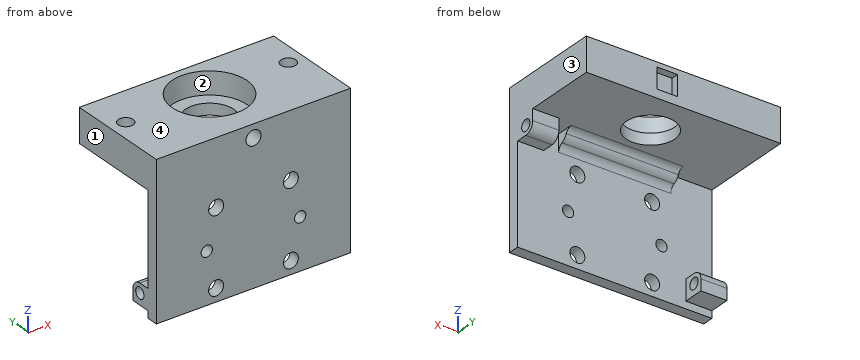
Autodesk Inventor part; units mm, degrees
ref_plane "YZ Plane" through (0, 0, 0) normal (1, 0, 0) x (0, 1, 0)
ref_plane "XZ Plane" through (0, 0, 0) normal (0, 1, 0) x (-1, 0, 0)
ref_plane "XY Plane" through (0, 0, 0) normal (0, 0, 1) x (1, 0, 0)
sketch "Boceto1" plane through (0, 0, 0) normal (0, 0, 1) x (1, 0, 0)
  line L0 (-26, 1.5) -> (26, 1.5)
  line L1 (26, 1.5) -> (26, -1.5)
  line L2 (26, -1.5) -> (-26, -1.5)
  line L3 (-26, -1.5) -> (-26, 1.5)
  line L4 (2.9301, 0) -> (0, 0)
  line L5 (0, 0) -> (0, 1.8389)
  dimension "d0" = 52
  dimension "d1" = 3
extrude "Extrusión1" add sketch "Boceto1" along normal blind 30
sketch "Boceto3" plane through (-26, 1.5, 0) normal (0, 1, 0) x (1, 0, 0)
  line L0 (52, 0) -> (52, -30)
  line L1 (0, -30) -> (52, -30)
  line L2 (52, 0) -> (47, 0)
  line L3 (47, 0) -> (47, -30)
  line L4 (47, -30) -> (52, -30)
  line L5 (52, -30) -> (52, 0)
  line L6 (0, 0) -> (0, -30)
  line L7 (0, 0) -> (5, 0)
  line L8 (5, 0) -> (5, -30)
  line L9 (5, -30) -> (0, -30)
  line L10 (0, -30) -> (0, 0)
  point P0 (26, 0)
  point P1 (5, -30)
  dimension "d4" = 5
  dimension "d5" = 5
extrude "Extrusión2" add sketch "Boceto3" along normal blind 25
sketch "Boceto5" plane through (0, 0, 30) normal (0, 0, 1) x (1, 0, 0)
  line L0 (-26, -1.5) -> (26, -1.5)
  line L1 (-26, -1.5) -> (-26, 26.5)
  line L2 (26, -1.5) -> (-26, -1.5)
  line L3 (-26, -1.5) -> (-26, 26.5)
  line L4 (-26, 26.5) -> (26, 26.5)
  line L5 (26, 26.5) -> (26, -1.5)
  point P0 (0, 0)
extrude "Extrusión4" add sketch "Boceto5" along normal blind 3
sketch "Boceto6" plane through (0, 0, 33) normal (0, 0, 1) x (1, 0, 0)
  circle A0 centre (0, 14.5) radius 6.5
  line L0 (26, -1.5) -> (26, 26.5)
  line L1 (26, 26.5) -> (-26, 26.5)
  line L2 (-26, 26.5) -> (-26, -1.5)
  point P0 (0, 0)
  point P1 (2.0533, 26.5)
  point P2 (-6.2533, 26.5)
  dimension "d12" = 13
  dimension "d13" = 26
  dimension "d14" = 12
  dimension "d38" = 52
extrude "Extrusión5" cut sketch "Boceto6" against normal up to surface (3 mm away)
sketch "Boceto7" plane through (-21, 1.5, 0) normal (0, 1, 0) x (1, 0, 0)
  circle A0 centre (33.5, -11.5916) radius 1.5
  circle A1 centre (8.5, -11.5916) radius 1.5
  line L0 (21, 0) -> (21, -4.282)
  line L1 (47, -33) -> (-5, -33)
  dimension "d17" = 25
  dimension "d18" = 12.5
  dimension "d19" = 3
  dimension "d20" = 3
  dimension "d68" = 21.4084
extrude "Extrusión6" cut sketch "Boceto7" against normal through all
sketch "Boceto9" plane through (0, 0, 33) normal (0, 0, 1) x (1, 0, 0)
  circle A0 centre (0, 14.5) radius 6.5
  line L0 (-26, 26.5) -> (-26, -1.5)
  line L1 (26, 26.5) -> (-26, 26.5)
  line L2 (26, -1.5) -> (26, 26.5)
  line L3 (-26, -1.5) -> (26, -1.5)
  circle A1 centre (0, 14.5) radius 10
  point P0 (0, 0)
  point P1 (0, 26.5)
  dimension "d32" = 20
extrude "Extrusión8" add sketch "Boceto9" along normal blind 6 contours L1 L2 L3 L0
sketch "Boceto8" plane through (0, 0, 39) normal (0, 0, 1) x (1, 0, 0)
  circle A0 centre (21.75, 15.395) radius 2
  circle A1 centre (-21.75, 15.395) radius 2
  line L0 (26, 26.5) -> (-26, 26.5)
  circle A2 centre (0, 14.5) radius 10
  point P0 (0, 0)
  dimension "d23" = 4
  dimension "d24" = 4
  dimension "d25" = 43.5
  dimension "d35" = 11.105
  dimension "d36" = 11.105
  dimension "d37" = 21.75
extrude "Extrusión7" cut sketch "Boceto8" against normal blind 5 contours A0 | A1
sketch "Boceto10" plane through (-26, 26.5, 0) normal (0, 1, 0) x (1, 0, 0)
  circle A0 centre (30.3, -35) radius 2
  line L0 (52, 0) -> (52, -39)
  line L1 (52, -39) -> (0, -39)
  line L2 (27.55, -32.25) -> (33.05, -32.25)
  line L3 (33.05, -32.25) -> (33.05, -37.75)
  line L4 (33.05, -37.75) -> (27.55, -37.75)
  line L5 (27.55, -37.75) -> (27.55, -32.25)
  line L6 (27.55, -32.25) -> (33.05, -37.75) construction
  line L7 (33.05, -32.25) -> (27.55, -37.75) construction
  point P0 (26, 0)
  dimension "d39" = 21.7
  dimension "d41" = 4
  dimension "d45" = 5.5
  dimension "d46" = 5.5
extrude "Extrusión9" cut sketch "Boceto10" against normal blind 2 contours A0 | L2 L3 L4 L5
sketch "Boceto11" plane through (26, -1.5, 0) normal (1, 0, 0) x (0, 0, -1)
  line L0 (-30, 28) -> (0, 28)
  line L1 (0, 28) -> (-30, 28)
  line L2 (-30, 28) -> (-30, 3)
  line L3 (-30, 3) -> (0, 3)
  line L4 (0, 3) -> (0, 28)
  point P0 (0, 1.5)
  dimension "d47" = 30
  dimension "d48" = 25
extrude "Extrusión10" cut sketch "Boceto11" against normal up to surface (52 mm away)
sketch "Boceto12" plane through (-26, -1.5, 0) normal (0, -1, 0) x (1, 0, 0)
  circle A0 centre (26, 35.5) radius 2
  line L0 (0, 0) -> (0, 39)
  line L1 (52, 0) -> (52, 39)
  line L2 (0, 39) -> (52, 39)
  point P0 (26, 0)
  dimension "d51" = 4
  dimension "d52" = 52
  dimension "d53" = 26
  dimension "d54" = 3.5
extrude "Extrusión11" cut sketch "Boceto12" against normal blind 5
sketch "Boceto13" plane through (26, -1.5, 0) normal (1, 0, 0) x (0, 0, -1)
  line L0 (-30, 3) -> (0, 3)
  line L1 (-24.5, 3) -> (-24.5, 8.5)
  line L2 (-24.5, 3) -> (-19, 3) construction
  line L3 (-24.5, 8.5) -> (-30, 8.5)
  line L4 (-30, 3) -> (-30, 28)
  circle A0 centre (-27, 6) radius 1.5
  point P0 (0, 1.5)
  dimension "d57" = 5.5
  dimension "d58" = 90
  dimension "d59" = 5.5
  dimension "d63" = 3
  dimension "d64" = 3
  dimension "d65" = 3
extrude "Extrusión12" add sketch "Boceto13" against normal blind 7
fillet "Empalme2" radius 2.5 1 edges at (22.5, 7, 24.5)
sketch "Boceto16" plane through (-26, 1.5, 0) normal (0, 1, 0) x (1, 0, 0)
  line L0 (0, -30) -> (0, 0)
  line L1 (0, 0) -> (52, 0)
  line L2 (52, 0) -> (52, 1.908)
  line L3 (52, 1.908) -> (0, 1.908)
  line L4 (0, 1.908) -> (0, 0)
  line L5 (52, 0) -> (52, -24.5)
  point P0 (26, 0)
  dimension "d69" = 1.908
extrude "Extrusión13" add sketch "Boceto16" against normal up to surface (3 mm away)
sketch "Boceto17" plane through (-26, 1.5, 30) normal (0, 1, 0) x (1, 0, 0)
  circle A0 centre (16, 28.408) radius 2
  line L0 (52, 31.908) -> (0, 31.908)
  point P0 (26, 30)
  dimension "d72" = 4
  dimension "d73" = 3.5
  dimension "d82" = 10
extrude "Extrusión14" cut sketch "Boceto17" against normal through all
pattern_linear "Patrón rectangular1" count 2 spacing 20 along (1, 0, 0) count 2 spacing 20 along (0, 0, 1) of "Extrusión14"
sketch "Boceto18" plane through (0, 0, 0) normal (1, 0, 0) x (0, 1, 0)
  line L0 (26.5, 30) -> (1.5, 30)
  line L1 (1.5, -1.908) -> (1.5, 30)
  arc A0 (1.5, 27) -> (4.5, 30) centre (1.5, 30) ccw
  point P0 (0, 0)
  point P1 (4.5, 30)
  dimension "d83" = 3
extrude "Extrusión15" add sketch "Boceto18" along normal mid plane 30
fillet "Empalme3" radius 2 2 edges at (0, 1.5, 27) (0, 4.5, 30)
sketch "Boceto19" plane through (-26, 1.5, 30) normal (-1, 0, 0) x (0, 0, 1)
  line L0 (-5.5, 0) -> (-31.908, 0)
  line L1 (-24.5, 0) -> (-30, 0)
  line L2 (-30, 0) -> (-30, 5.5)
  line L3 (-30, 5.5) -> (-24.5, 5.5)
  line L4 (-24.5, 5.5) -> (-24.5, 0)
  line L5 (0, 25) -> (0, 0)
  circle A0 centre (-27, 3) radius 1.5
  point P0 (-30, -1.5)
  point P1 (-30, 0)
  dimension "d87" = 5.5
  dimension "d88" = 5.5
  dimension "d89" = 24.5
  dimension "d93" = 3
  dimension "d94" = 3
  dimension "d95" = 2.5
extrude "Extrusión16" add sketch "Boceto19" against normal blind 7
fillet "Empalme4" radius 2.5 1 edges at (-22.5, 7, 5.5)
equation "\"d13\" = 0.5 * d38"
equation "\"d18\" = 0.5 * d17"
equation "\"d20\" = d19"
equation "\"d24\" = d23"
equation "\"d36\" = d35"
equation "\"d53\" = 0.5 * d52"
equation "\"d59\" = d57"
properties part number "Soporte Extruder Izq" material "Polipropileno"
Design review of the part built by this model. Coordinates are the model's own, in mm. Face numbers are marked on the shaded views. Give positions to 0.01 mm unless a question says otherwise; leave off trailing zeros. Loops run counter-clockwise (first coordinate to the right, second up) from the corner with the lowest first, then second, coordinate; pieces in that order, holes last. Notation, with made-up numbers: M 60,80 L 75,80 A18 ccw 75,88 Z; hole C 86.25,27.5 d1. An arc over 180 degrees is marked long. Return JSON: item names as keys, results as strings. Group by question number.
Item 1: We need section B-B (z = 11). Give the boundary of the cut face in (x, y), and give its area (3 significant figures).
Item 2: We need section D-D (x = 21.75). Give the boundary of the cut face in (y, z) (3 decimals).
Item 3: Insertion check: pin 1 Ø1.2 at (x, y) = (-22.5, 15) entering from +Z; pin 2 Ø10 at (x, y) = (-5, 14) entering from -Z; pin 3 Ø0.9 at (x, y) = (22, 3.5) entering from -Z. Each pin has a flat end and moves straight along its axis. Give the tip position at first contact, or say it passes through.
Item 4: Mouldability with a two-part tool opening along X and no side actions: class the marked faces 1, 2, 3 and 4 as released by +X, released by -X, zero draft, split by the parting line, or undercut.
Item 5: For probe 1 along Z at (x, y) = (10, 0.5); probe 2 along Z at (x, y) = (-12.5, -0.15); probe 3 along Y at (x, z) = (-20.75, 3), list the stretches that pass through material, from the lowest coordinate up.
Item 6: We need section C-C (y = 14.5). Give the boundary of the cut face in (x, z).
Item 7: We need section A-A (x = 0). Give the boundary of the cut face in (y, z).
Output:
{
 "1": {"outline": "M -26,-1.5 L -13.88,-1.5 L -13.88,1.5 L -26,1.5 Z; M -11.12,-1.5 L 11.12,-1.5 L 11.12,1.5 L -11.12,1.5 Z; M 13.88,-1.5 L 26,-1.5 L 26,1.5 L 13.88,1.5 Z", "area": "139 mm^2"},
 "2": {"outline": "M -1.5,-1.908 L 1.5,-1.908 L 1.5,24.5 L 4.5,24.5 A2.5 ccw 7,27 L 7,30 L 26.5,30 L 26.5,39 L 17.395,39 L 17.395,34 L 13.395,34 L 13.395,39 L -1.5,39 Z; hole C 4.5,27 d3"},
 "3": {"pin 1": "stops at z = 34", "pin 2": "stops at z = 30", "pin 3": "stops at z = 24.5"},
 "4": {"face 1": "released by -X", "face 2": "undercut", "face 3": "released by +X", "face 4": "zero draft"},
 "5": {"probe 1": "z = -1.91 to -0.41, 3.59 to 19.59, 23.59 to 39", "probe 2": "z = -1.91 to 10.09, 13.09 to 39", "probe 3": "y = -1.5 to 3, 6 to 7"},
 "6": {"outline": "M -26,30 L -6.5,30 L -6.5,33 L -10,33 L -10,39 L -19.96,39 L -19.96,34 L -23.54,34 L -23.54,39 L -26,39 Z; M 6.5,30 L 26,30 L 26,39 L 23.54,39 L 23.54,34 L 19.96,34 L 19.96,39 L 10,39 L 10,33 L 6.5,33 Z"},
 "7": {"outline": "M -1.5,-1.91 L 1.5,-1.91 L 1.5,25.42 A2 cw 2.7,27.25 A3 ccw 4.25,28.8 A2 cw 6.08,30 L 8,30 L 8,33 L 4.5,33 L 4.5,39 L -1.5,39 L -1.5,37.5 L 3.5,37.5 L 3.5,33.5 L -1.5,33.5 Z; M 21,30 L 26.5,30 L 26.5,39 L 24.5,39 L 24.5,33 L 21,33 Z"}
}
